Can you work these out from the model? Positions are in its coordinate system, mm. A direction names the side the tool comes from. Give positions to 0.01 mm unless a question says otherwise; leave off trailing zeros. Loops run counter-clockwise (first coordinate to the right, second up) from the corner with the lowest first, then second, coordinate; pieces in that order, holes last. Notation, with made-up numbers: (-18.5, 19) - (8.5, 19) arc R18 cw to (8.5, 41) - close; hole circle Ø3 at (4.5, 15). An arc over 180 degrees is marked (long way). Answer as a JSON object with one key per item and string values. Group by question number.
Item 1: Suppose I cut it at C-C on x = 30. Write out the boundary of the cut face in (y, z).
Item 2: Thinking about a two-plate mould opening in X: for faces 1 (the flat face through (9, 13, -20)), 2 (the flat face through (18, 15.4, -12.4)), 3 (the flat face through (25.4, 1, -1.8)), which applies, pulls with the +X half, pulls with the -X half, needs draft (parallel to the pull), parting line crosses it, or undercut?
Item 3: Will these pins go through, and if not, where does the flat tip stop? pin 1 (4.5 mm diameter, centred on x = 30, y = 15.5, fed in from +Z); pin 2 (6 mm diameter, centred on x = 50, z = -10, fed in from +Y); pin 3 (4.5 mm diameter, centred on y = 13, z = -21.5, fed in from -X).
Item 4: Suppose I cut it at A-A on x = 50. Write out the boundary of the cut face in (y, z), and give its area (3 significant figures).
Item 5: Please list where these lines run through material, in increasing order: L1, parallel to X at y = 1.5, z = -10; L2, parallel to X at y = 11.5, z = -7.25; L3, parallel to Z at x = 49, y = 4.5.
Item 6: Which directions (+Z, -Z, +X, -X, +Y, -Y) give clear straight access to the entire face, cutting with the end or side of a thin tool? Please do faces 4 (the flat face through (34.6, 1, -18.2)), 5 (the flat face through (42, 17, -10)), 6 (the flat face through (34.7, 1, -1.7)), 7 (the flat face through (37, 12.8, -12.4)).
Item 7: Suppose I cut it at B-B on z = -22. Write out the boundary of the cut face in (x, y), and give its area (3 significant figures).
Item 8: Suppose I cut it at D-D on y = 4. Write out the boundary of the cut face in (x, z).
from build123d import *

# Parameters (mm, degrees)
SKETCH1_W           = 60
SKETCH1_H           = 20
SKETCH1_R           = 2.5
BOSS_EXTRUDE1_DEPTH = 2
FILLET1_SIZE        = 0.7
CUT_EXTRUDE2_DEPTH  = 2
BOSS_EXTRUDE3_DEPTH = 22
BOSS_EXTRUDE4_DEPTH = 24
CUT_EXTRUDE3_DEPTH  = 24
SKETCH6_R           = 2.5
CUT_EXTRUDE4_DEPTH  = 55.45181356
FILLET2_R           = 10
FILLET4_R           = 5
CHAMFER1_SIZE       = 0.7


with BuildPart() as part:
    # Sketch1 → Boss-Extrude1 (new body)
    with BuildSketch(Plane(origin=(0, 0, 0), x_dir=(1, 0, 0), z_dir=(0, 1, 0))):
        with Locations((30, 10)):
            Rectangle(SKETCH1_W, SKETCH1_H)
        with Locations(Location((10, 10, 0), (0, 0, 270))):
            Circle(SKETCH1_R, mode=Mode.SUBTRACT)
        with Locations(Location((30, 10, 0), (0, 0, 270))):
            Circle(SKETCH1_R, mode=Mode.SUBTRACT)
        with Locations(Location((50, 10, 0), (0, 0, 270))):
            Circle(SKETCH1_R, mode=Mode.SUBTRACT)
    extrude(amount=BOSS_EXTRUDE1_DEPTH)

    # Fillet1
    fillet1_edges = [part.edges().sort_by_distance(p)[0] for p in [
        (0, 1, -20),
        (60, 1, -20),
        (60, 1, 0),
        (0, 1, 0),
    ]]
    chamfer(fillet1_edges, length=FILLET1_SIZE)

    # Sketch2 → Cut-Extrude2 (cut)
    with BuildSketch(Plane(origin=(0, 2, 0), x_dir=(1, 0, 0), z_dir=(0, 1, 0))):
        Polygon((30, 20), (30, 16.5), (32.9, 16.5), (36.4, 20), (32.9, 20), align=None)
        Polygon((27.1, 16.5), (30, 16.5), (30, 20), (27.1, 20), (23.6, 20), align=None)
        Polygon((30, 0), (30, 3.5), (27.1, 3.5), (23.6, 0), (27.1, 0), align=None)
        Polygon((32.9, 3.5), (30, 3.5), (30, 0), (32.9, 0), (36.4, 0), align=None)
    extrude(amount=-CUT_EXTRUDE2_DEPTH, mode=Mode.SUBTRACT)

    # Sketch3 → Boss-Extrude3 (add)
    with BuildSketch(Plane(origin=(0, 2, 0), x_dir=(1, 0, 0), z_dir=(0, 1, 0))):
        Polygon((23, 0), (23, 10), (23, 20), (18, 20), (18, 0), align=None)
        Polygon((37, 20), (37, 10), (37, 0), (42, 0), (42, 20), align=None)
    extrude(amount=BOSS_EXTRUDE3_DEPTH)

    # Sketch4 → Boss-Extrude4 (add)
    with BuildSketch(Plane(origin=(0, 0, 0), x_dir=(1, 0, 0), z_dir=(0, 1, 0))):
        Polygon((0.7, 20), (0.7, 25), (59.3, 25), (59.3, 20), (23.6, 20), align=None)
    extrude(amount=BOSS_EXTRUDE4_DEPTH)

    # Sketch5 → Cut-Extrude3 (cut)
    with BuildSketch(Plane(origin=(0, 24, 0), x_dir=(1, 0, 0), z_dir=(0, 1, 0))):
        Polygon((23.6, 20), (27.100178567, 23.500178567), (32.900178567, 23.500178567), (36.4, 20), align=None)
    extrude(amount=-CUT_EXTRUDE3_DEPTH, mode=Mode.SUBTRACT)

    # Sketch6 → Cut-Extrude4 (cut, through all)
    with BuildSketch(Plane(origin=(42, 0, 0), x_dir=(0, 0, -1), z_dir=(1, 0, 0))):
        with Locations((10, 14)):
            Circle(SKETCH6_R)
    extrude(amount=-CUT_EXTRUDE4_DEPTH, mode=Mode.SUBTRACT)

    # Fillet2
    fillet2_edges = [part.edges().sort_by_distance(p)[0] for p in [
        (20.5, 24, 0),
        (39.5, 24, 0),
    ]]
    fillet(fillet2_edges, radius=FILLET2_R)

    # Fillet4
    fillet4_edges = [part.edges().sort_by_distance(p)[0] for p in [
        (18, 2, -10),
        (42, 2, -10),
    ]]
    fillet(fillet4_edges, radius=FILLET4_R)

    # Chamfer1
    chamfer1_edges = [part.edges().sort_by_distance(p)[0] for p in [
        (59.3, 12, -25),
        (0.7, 12, -25),
    ]]
    chamfer(chamfer1_edges, length=CHAMFER1_SIZE)


solid = part.part
Worked out:
{
 "1": {"outline": "(0, -25) - (24, -25) - (24, -23.5) - (0, -23.5) - close; (0, -16.5) - (2, -16.5) - (2, -12.5) - (0, -12.5) - close; (0, -7.5) - (2, -7.5) - (2, -3.5) - (0, -3.5) - close"},
 "2": {"face 1": "needs draft", "face 2": "pulls with the -X half", "face 3": "undercut"},
 "3": {"pin 1": "stops at z = -23.5", "pin 2": "stops at y = 2", "pin 3": "stops at x = 0.7"},
 "4": {"outline": "(0, -25) - (24, -25) - (24, -20) - (2, -20) - (2, -12.5) - (0, -12.5) - close; (0, -7.5) - (2, -7.5) - (2, 0) - (0, 0) - close", "area": "150 mm2"},
 "5": {"L1": "x = 0 to 7.5, 12.5 to 27.5, 32.5 to 47.5, 52.5 to 60", "L2": "x = 18 to 23, 37 to 42", "L3": "z = -25 to -20"},
 "6": {"face 4": "+Y, -Y", "face 5": "+Z, +X, +Y", "face 6": "+Z, +Y, -Y", "face 7": "+Z, +Y"},
 "7": {"outline": "(0.7, 0) - (25.6, 0) - (25.6, 24) - (0.7, 24) - close; (34.4, 0) - (59.3, 0) - (59.3, 24) - (34.4, 24) - close", "area": "1,200 mm2"},
 "8": {"outline": "(0.7, -24.3) - (1.4, -25) - (58.6, -25) - (59.3, -24.3) - (59.3, -20) - (43, -20) - (43, 0) - (37, 0) - (37, -20) - (36.4, -20) - (32.9, -23.5) - (27.1, -23.5) - (23.6, -20) - (23, -20) - (23, 0) - (17, 0) - (17, -20) - (0.7, -20) - close"}
}
